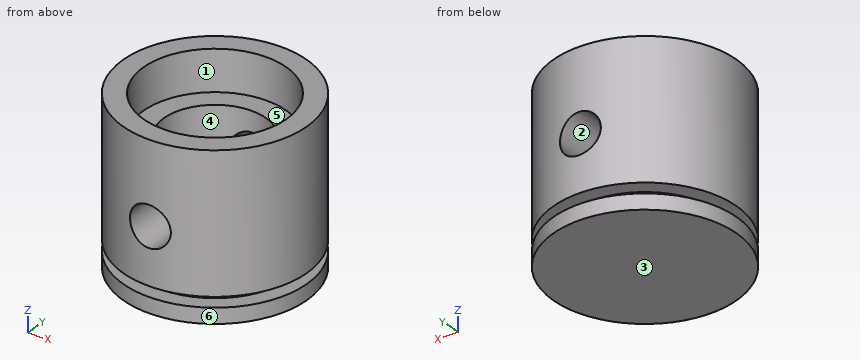
```python
from build123d import *

# Parameters (mm, degrees)
SKETCH1_R                                = 9
BOSS_EXTRUDE1_DEPTH                      = 16
CBORE_FOR_M14_HEX_HEAD_BOLT1_D           = 10
CBORE_FOR_M14_HEX_HEAD_BOLT1_DEPTH       = 14
CBORE_FOR_M14_HEX_HEAD_BOLT1_CBORE_D     = 14
CBORE_FOR_M14_HEX_HEAD_BOLT1_CBORE_DEPTH = 4
SKETCH4_R                                = 9
SKETCH4_R_2                              = 7.5
CUT_EXTRUDE1_DEPTH                       = 1
SKETCH5_R                                = 2
CUT_EXTRUDE2_DEPTH                       = 15.5


with BuildPart() as part:
    # Sketch1 → Boss-Extrude1 (new body)
    with BuildSketch(Plane.XY):
        Circle(SKETCH1_R)
    extrude(amount=BOSS_EXTRUDE1_DEPTH)

    # CBORE for M14 Hex Head Bolt1
    with Locations(Plane.XY.offset(16)):
        with Locations((0, 0)):
            CounterBoreHole(CBORE_FOR_M14_HEX_HEAD_BOLT1_D / 2, CBORE_FOR_M14_HEX_HEAD_BOLT1_CBORE_D / 2, CBORE_FOR_M14_HEX_HEAD_BOLT1_CBORE_DEPTH, depth=CBORE_FOR_M14_HEX_HEAD_BOLT1_DEPTH)

    # Sketch4 → Cut-Extrude1 (cut)
    with BuildSketch(Plane.XY.offset(2.5)):
        Circle(SKETCH4_R)
        Circle(SKETCH4_R_2, mode=Mode.SUBTRACT)
    extrude(amount=-CUT_EXTRUDE1_DEPTH, mode=Mode.SUBTRACT)

    # Sketch5 → Cut-Extrude2 (cut, symmetric)
    with BuildSketch(Plane(origin=(0, 0, 0), x_dir=(1, 0, 0), z_dir=(0, 1, 0))):
        with Locations(Location((0, -8, 0), (0, 0, 270))):  # turned: the seam where the file's is
            Circle(SKETCH5_R)
    extrude(amount=CUT_EXTRUDE2_DEPTH, both=True, mode=Mode.SUBTRACT)


solid = part.part
```
Could you check a few things on this model? Use its own coordinates, in mm. Face numbers are marked on the shaded views. A direction names the side the tool comes from. Coordinates: 2 decimals unless noted, no trailing zeros. Loops run counter-clockwise (first coordinate to the right, second up) from the corner with the lowest first, then second, coordinate; pieces in that order, holes last.
1) Please list where these lines run through material, in increasing order: line 1 along Z through (x, y) = (0, 6.35); line 2 along Y through (x, z) = (0.25, 3.25); line 3 along Y through (x, z) = (0, 13.8).
Reported:
line 1: z = 0 to 6, 10 to 12
line 2: y = -9 to -4.99, 4.99 to 9
line 3: y = -9 to -7, 7 to 9
2) Thinking about a two-plate mould opening in X: for the marked faces 3, 4, 5 and 6, which applies, released by +X, released by -X, zero draft, split by the parting line, or undercut?
Reported:
face 3: zero draft
face 4: undercut
face 5: undercut
face 6: split by the parting line
3) Imagine slicing it at D-D (z = 5.5). List the corners of the cut face in (x, y) for me, and give its area (3 significant figures).
Reported:
outline: circle Ø18 at (0, 0); hole circle Ø10 at (0, 0)
area: 176 mm2
4) Imagine slicing it at B-B (z = 8.75). List the corners of the cut face in (x, y) for me.
Reported:
outline: (-1.85, -8.81) - (-1.85, -4.64) arc R5 cw to (-1.85, 4.64) - (-1.85, 8.81) arc R9 ccw to start; (1.85, -8.81) arc R9 ccw to (1.85, 8.81) - (1.85, 4.64) arc R5 cw to (1.85, -4.64) - close
5) Will these pins go through, and if not, where does the flat tip stop? pin 1 Ø8 at (x, z) = (-3, 8) entering from -Y; pin 2 Ø5 at (x, y) = (-3, 3) entering from +Z; pin 3 Ø3 at (x, z) = (0, 8) entering from +Y; pin 4 Ø4 at (x, z) = (-2.5, 6) entering from +Y.
Reported:
pin 1: stops at y = -9
pin 2: stops at z = 12
pin 3: passes through
pin 4: stops at y = 8.99
6) Imagine slicing it at A-A (x = 0). List the corners of the cut face in (y, z) for me, and give its area (3 significant figures).
Reported:
outline: (-9, 0) - (9, 0) - (9, 1.5) - (7.5, 1.5) - (7.5, 2.5) - (9, 2.5) - (9, 6) - (5, 6) - (5, 2) - (-5, 2) - (-5, 6) - (-9, 6) - (-9, 2.5) - (-7.5, 2.5) - (-7.5, 1.5) - (-9, 1.5) - close; (-9, 10) - (-5, 10) - (-5, 12) - (-7, 12) - (-7, 16) - (-9, 16) - close; (5, 10) - (9, 10) - (9, 16) - (7, 16) - (7, 12) - (5, 12) - close
area: 97.0 mm2
7) Imagine slicing it at C-C (y = 0). List the corners of the cut face in (x, z) for me, and give its area (3 significant figures).
Reported:
outline: (-9, 0) - (9, 0) - (9, 1.5) - (7.5, 1.5) - (7.5, 2.5) - (9, 2.5) - (9, 16) - (7, 16) - (7, 12) - (5, 12) - (5, 2) - (-5, 2) - (-5, 12) - (-7, 12) - (-7, 16) - (-9, 16) - (-9, 2.5) - (-7.5, 2.5) - (-7.5, 1.5) - (-9, 1.5) - close
area: 129 mm2
8) Which directions (+Z, -Z, +X, -X, +Y, -Y) give clear straight access to the entire face, cutting with the end or side of a thin tool? Please do the marked faces 1 and 2.
Reported:
face 1: +Z
face 2: +Y, -Y
